Verification items for the finished model (mm, model axes). Face numbers are marked on the shaded views. Coordinates: 2 decimals unless noted, no trailing zeros. Order: outer loops, then holes, each group sorted by start corner. A loop starts at its lowest first (then second) coordinate and runs counter-clockwise, first axis right, second up. Notation, with made-up numbers: (48, -13) -> (100, -13) arc R20 ccw to (100, 22) -> close; hole circle Ø7 at (44, -19.75). An arc over 180 degrees is marked (long way). Write item = value, one per line. Start each with the question number.
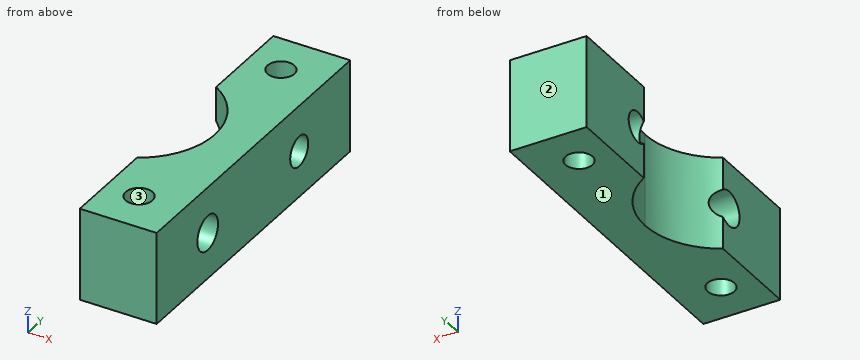
from build123d import *

# Parameters (mm, degrees)
F0_R     = 1.75
F1_DEPTH = 12
F2_R     = 1.96967
F2_R_2   = 2.258854
F3_DEPTH = 25


with BuildPart() as f1:
    # F0 (on Top) → F1 (new body)
    with BuildSketch(Plane.XY):
        with BuildLine():
            ThreePointArc((-10, 29.810254), (-6.339746, 26.15), (-5, 21.15))
            ThreePointArc((-5, 21.15), (-6.339746, 16.15), (-10, 12.489746))
            Line((-10, 12.489746), (-10, 0))
            Line((-10, 0), (0, 0))
            Line((0, 0), (0, 42.3))
            Line((0, 42.3), (-10, 42.3))
            Line((-10, 42.3), (-10, 29.810254))
        make_face()
        with Locations((-5.65, 5.65)):
            Circle(F0_R, mode=Mode.SUBTRACT)
        with Locations((-5.65, 36.65)):
            Circle(F0_R, mode=Mode.SUBTRACT)
    extrude(amount=F1_DEPTH)

    # F2 (on face) → F3 (cut)
    with BuildSketch(Plane.YZ):
        with Locations((31.15, 6)):
            Circle(F2_R)
        with Locations((11.15, 6)):
            Circle(F2_R_2)
    extrude(amount=-F3_DEPTH, mode=Mode.SUBTRACT)


solid = f1.part
Item 1: Gauge pin test, flat end, axial feed: P1, Ø4, axis at x = -4, y = 26.5, coming from the -Z side. Record the tip position at first contact, or that the pin passes through.
Item 2: Section check B-B (z = 5.5). Record the boundary of the cut face in (x, y).
Item 3: Mould release check, pull along Y, two halves, no side actions. Record for the marked faces 1, 2 and 3: pulls with the +Y half, pulls with the -Y half, needs draft (parallel to the pull), parting line crosses it, or undercut.
Item 4: Section check A-A (y = 11.15). Record the boundary of the cut face in (x, z), then the cut area to 3 significant figures.
Item 5: Section check C-C (x = -6.5). Record the boundary of the cut face in (y, z), then the cut area to 3 significant figures.
Item 6: Section check D-D (x = -2). Record the boundary of the cut face in (y, z), then the cut area to 3 significant figures.
Item 7: Thickness scan on line 1 (Z direction, x = -2.75, y = 11.15); line 2 (Y direction, x = -6, z = 2.25); line 3 (Y direction, x = -6.75, z = 10.75). Record the ranges inside material, lowest first.
Filled sheet:
q1.P1 = 0
q2.outline = (-10, 0) -> (0, 0) -> (0, 8.95) -> (-10, 8.95) -> close; (-10, 33.06) -> (0, 33.06) -> (0, 42.3) -> (-10, 42.3) -> close; (-9.13, 29.24) arc R10 cw to (-8.74, 13.35) -> (0, 13.35) -> (0, 29.24) -> close; hole circle Ø3.5 at (-5.65, 5.65); hole circle Ø3.5 at (-5.65, 36.65)
q3.face_1 = needs draft
q3.face_2 = pulls with the +Y half
q3.face_3 = undercut
q4.outline = (-10, 0) -> (0, 0) -> (0, 3.74) -> (-10, 3.74) -> close; (-10, 8.26) -> (0, 8.26) -> (0, 12) -> (-10, 12) -> close
q4.area = 74.8 mm^2
q5.outline = (0, 0) -> (4.12, 0) -> (4.12, 12) -> (0, 12) -> close; (7.18, 0) -> (15.88, 0) -> (15.88, 12) -> (7.18, 12) -> close; (26.42, 0) -> (35.12, 0) -> (35.12, 12) -> (26.42, 12) -> close; (38.18, 0) -> (42.3, 0) -> (42.3, 12) -> (38.18, 12) -> close; hole circle Ø4.52 at (11.15, 6); hole circle Ø3.94 at (31.15, 6)
q5.area = 280 mm^2
q6.outline = (0, 0) -> (42.3, 0) -> (42.3, 12) -> (0, 12) -> close; hole circle Ø4.52 at (11.15, 6); hole circle Ø3.94 at (31.15, 6)
q6.area = 479 mm^2
q7.line_1 = 0 to 3.74, 8.26 to 12
q7.line_2 = 0 to 3.94, 7.36 to 16.79, 25.51 to 34.94, 38.36 to 42.3
q7.line_3 = 0 to 4.29, 7.01 to 15.5, 26.8 to 35.29, 38.01 to 42.3
